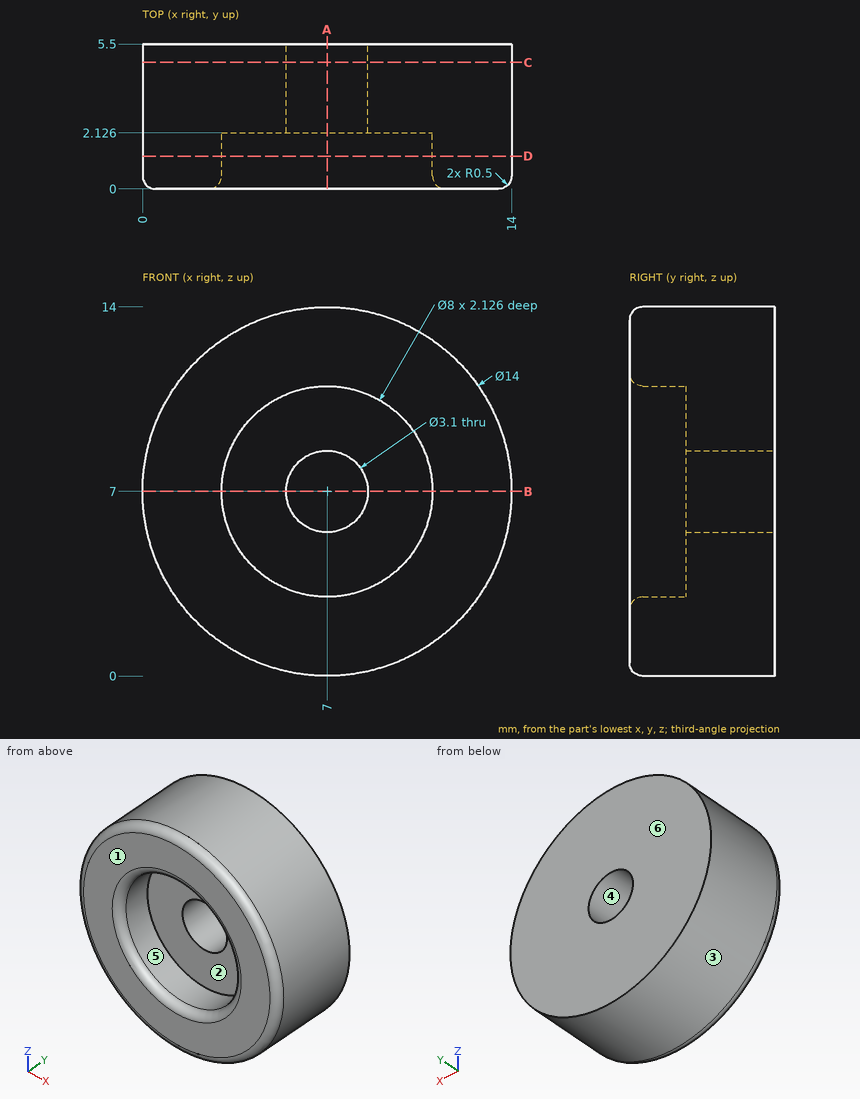
The figure shows three views and two pictorial views of one solid part (mm, origin at its lowest corner). Answer the questions. A direction names the side the tool comes from. Coordinates: 2 decimals unless noted, no trailing zeros. Write each loop counter-clockwise with the first axis right and the second up, starting at its lowest first coordinate (ties: lowest second). Pieces come first, ordered by that corner, then holes. Notation, with made-up numbers: (16, 37) -> (23, 37) arc R22 cw to (23, 48) -> close; hole circle Ø6 at (8, 16). An arc over 180 degrees is marked (long way). Return JSON: item names as keys, results as strings.
(1) For a pull along Z with two mould halves and no side action, classify the marked faces 3, 4, 5 and 6 as pulls with the +Z half, pulls with the -Z half, needs draft (parallel to the pull), parting line crosses it, or undercut.
Answers below:
{"face 3": "parting line crosses it", "face 4": "undercut", "face 5": "undercut", "face 6": "needs draft"}
(2) Which of the six approach directions +Z, -Z, +X, -X, +Y, -Y give full straight-line access (tool end or side, diameter ignored) to the marked faces 1 and 2?
Answers below:
{"face 1": "+Z, -Z, +X, -X, -Y", "face 2": "-Y"}
(3) The part is cut by section A-A on x = 7. Give the vertices of the cut face in (y, z).
Answers below:
{"outline": "(0, 0.5) arc R0.5 ccw to (0.5, 0) -> (5.5, 0) -> (5.5, 5.45) -> (2.13, 5.45) -> (2.13, 3) -> (0.5, 3) arc R0.5 ccw to (0, 2.5) -> close; (0, 11.5) arc R0.5 ccw to (0.5, 11) -> (2.13, 11) -> (2.13, 8.55) -> (5.5, 8.55) -> (5.5, 14) -> (0.5, 14) arc R0.5 ccw to (0, 13.5) -> close"}
(4) The part is cut by section D-D on y = 1.25. Give the vertices of the cut face in (x, z).
Answers below:
{"outline": "circle Ø14 at (7, 7); hole circle Ø8 at (7, 7)"}
(5) The part is cut by section B-B on z = 7. Give the vertices of the cut face in (x, y), then the cut area to 3 significant figures.
Answers below:
{"outline": "(0, 0.5) arc R0.5 ccw to (0.5, 0) -> (2.5, 0) arc R0.5 ccw to (3, 0.5) -> (3, 2.13) -> (5.45, 2.13) -> (5.45, 5.5) -> (0, 5.5) -> close; (8.55, 2.13) -> (11, 2.13) -> (11, 0.5) arc R0.5 ccw to (11.5, 0) -> (13.5, 0) arc R0.5 ccw to (14, 0.5) -> (14, 5.5) -> (8.55, 5.5) -> close", "area": "49.3 mm^2"}
(6) The part is cut by section C-C on y = 4.8. Give the vertices of the cut face in (x, z), then the cut area to 3 significant figures.
Answers below:
{"outline": "circle Ø14 at (7, 7); hole circle Ø3.1 at (7, 7)", "area": "146 mm^2"}
(7) Consider line 1 along Z through (x, y) = (7, 1.85); line 2 along Z through (x, y) = (7, 3.35); line 3 along Y through (x, z) = (6.25, 8.75). Determine where each line is inside the solid, lowest interval first. Write a range as from..to.
Answers below:
{"line 1": "0..3, 11..14", "line 2": "0..5.45, 8.55..14", "line 3": "2.13..5.5"}
(8) Each of these flat-tipped pins is pushed along its axis until it touches: P1, Ø2, axis at x = 12.5, z = 12.5, coming from the -Y side (1 decimal); P2, Ø1, axis at x = 12, z = 6.5, coming from the -Y side; P3, Ø1, axis at y = 1, z = 4.5, coming from the +X side. Where does it stop, or does it pass through?
Answers below:
{"P1": "y = 0.1", "P2": "y = 0", "P3": "x = 13.71"}
